Work out the finished part from the listing and answer in its coordinate system (mm). Give positions to 0.01 mm unless a question says otherwise; leave off trailing zeros. Loops run counter-clockwise (first coordinate to the right, second up) from the corner with the lowest first, then second, coordinate; pieces in that order, holes last. Notation, with made-up numbers: (23, -26) - (54, -26) arc R13 ccw to (54, -9) - close; hole circle Ø3 at (53, -27). An arc over 180 degrees is marked (long way). One line per question, with ' | ' between items. Start each with the question number.
1. Each of these flat-tipped pins is pushed along its axis until it touches: pin 1 (2 mm diameter, centred on x = -3, z = 2.5, fed in from -Y); pin 2 (4 mm diameter, centred on x = -1.5, z = 19.5, fed in from -Y); pin 3 (4 mm diameter, centred on x = -1, z = 31, fed in from +Y). Where does it stop, or does it pass through?
2. Section A-A (z = 36.5) is taken. Determine the outline of the cut face in (x, y).
3. Find the intervals of material crossed by line 1 (Y direction, x = 0, z = 48); line 2 (Z direction, x = 3.25, y = -1); line 3 (X direction, y = -1, z = 40), in increasing order.
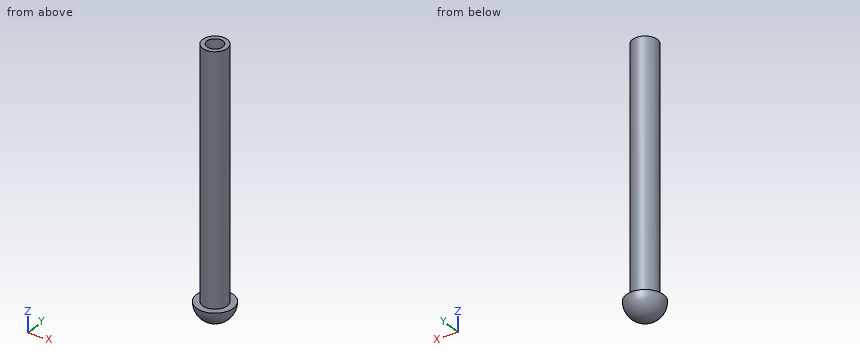
from build123d import *

# Parameters (mm, degrees)
F0_R     = 2.54
F1_DEPTH = 50.8
F3_R     = 1.651
F4_DEPTH = 6.35
F5_R     = 3.81
F6_DEPTH = 3.81
F7_R     = 3.80999


# Not quite as in the source:
# - a fillet or chamfer is up to 0.001 mm smaller than in the source, because OpenCascade refuses the exact size


with BuildPart() as f1:
    # F0 (on Top) → F1 (new body)
    with BuildSketch(Plane.XY):
        Circle(F0_R)
    extrude(amount=F1_DEPTH)

    # F3 (on face) → F4 (cut)
    with BuildSketch(Plane.XY.offset(50.8)):
        Circle(F3_R)
    extrude(amount=-F4_DEPTH, mode=Mode.SUBTRACT)

    # F5 (on face) → F6 (join)
    with BuildSketch(Plane(origin=(0, 0, 0), x_dir=(1, 0, 0), z_dir=(0, 0, -1))):
        Circle(F5_R)
    extrude(amount=F6_DEPTH)

    # F7 (radius 3.81 in the source; OpenCascade refuses exactly that, so slightly less here)
    f7_edges = [f1.edges().sort_by_distance(p)[0] for p in [
        (-3.81, 0, -3.81),
    ]]
    fillet(f7_edges, radius=F7_R)


solid = f1.part
Conclusion:
1) pin 1: y = -1.57 | pin 2: y = -2.54 | pin 3: y = 2.54
2) outline: circle Ø5.08 at (0, 0)
3) line 1: -2.54 to -1.65, 1.65 to 2.54 | line 2: -1.72 to 0 | line 3: -2.33 to 2.33
